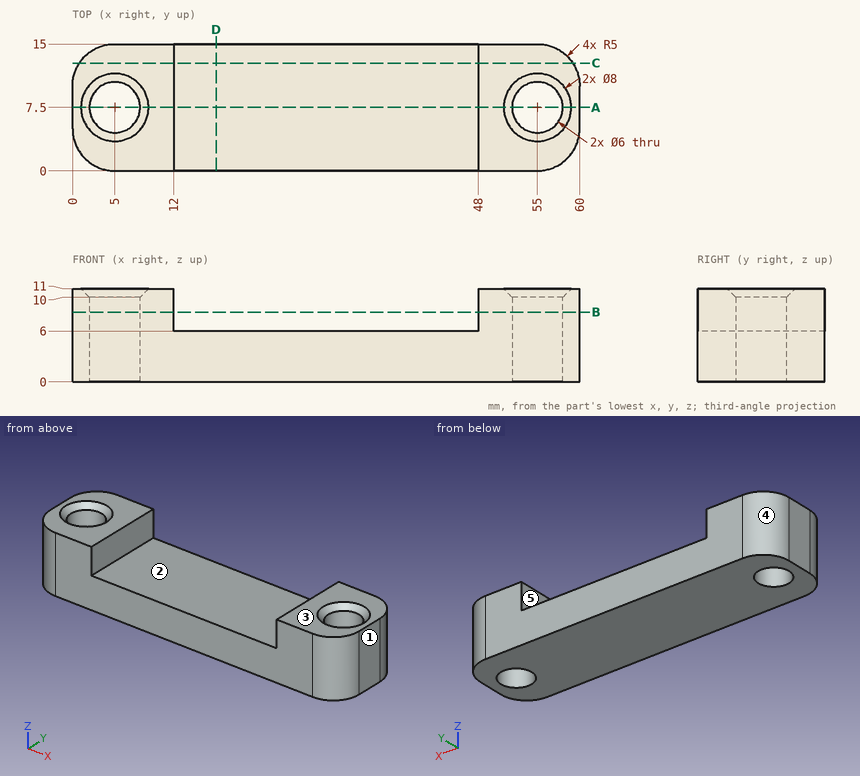
Answer from the drawing. Dimensions are ordinates in mm from the lowest x, y and z of the part. A direction names the side the tool comes from. Coordinates: 2 decimals unless noted, no trailing zeros. Loops run counter-clockwise (first coordinate to the right, second up) from the corner with the lowest first, then second, coordinate; pieces in that order, holes last. Notation, with made-up numbers: (87, -30.5) - (132, -30.5) arc R17 ccw to (132, -24.5) - close; hole circle Ø3 at (-36.75, -26). An arc over 180 degrees is marked (long way). Answer in a Markdown table with one row per item.
1. Find section D-D, the plane x = 17. Write down the section's boundary in (y, z), then the cut area to 3 significant figures.
Conclusion:
| item | result |
|---|---|
| outline | (0, 0) - (15, 0) - (15, 6) - (0, 6) - close |
| area | 90.0 mm² |
2. Find section B-B, the plane z = 8.25. Write down the section's boundary in (x, y), then the cut area to 3 significant figures.
Conclusion:
| item | result |
|---|---|
| outline | (0, 5) arc R5 ccw to (5, 0) - (12, 0) - (12, 15) - (5, 15) arc R5 ccw to (0, 10) - close; (48, 0) - (55, 0) arc R5 ccw to (60, 5) - (60, 10) arc R5 ccw to (55, 15) - (48, 15) - close; hole circle Ø6 at (5, 7.5); hole circle Ø6 at (55, 7.5) |
| area | 282 mm² |
3. Straight lines are drawn through the part: line 1 (X direction, y = 6, z = 7.5); line 2 (Z direction, x = 39.5, y = 1.5); line 3 (X direction, y = 9.5, z = 8). For each, find the intervals that lie inside material, in ascending order.
Conclusion:
| item | result |
|---|---|
| line 1 | x = 0 to 2.4, 7.6 to 12, 48 to 52.4, 57.6 to 60 |
| line 2 | z = 0 to 6 |
| line 3 | x = 0 to 2.76, 7.24 to 12, 48 to 52.76, 57.24 to 60 |
4. Find section C-C, the plane y = 12.75. Write down the section's boundary in (x, z), then the cut area to 3 significant figures.
Conclusion:
| item | result |
|---|---|
| outline | (0.82, 0) - (59.18, 0) - (59.18, 11) - (48, 11) - (48, 6) - (12, 6) - (12, 11) - (0.82, 11) - close |
| area | 462 mm² |
5. Determine the mould class of the marked faces 3, 4 and 5 for opening direction X: +X half, -X half, draft (parallel to the pull), parting line (faces both ways), or undercut.
Conclusion:
| item | result |
|---|---|
| face 3 | draft |
| face 4 | -X half |
| face 5 | undercut |
6. Find section A-A, the plane y = 7.5. Write down the section's boundary in (x, z).
Conclusion:
| item | result |
|---|---|
| outline | (0, 0) - (2, 0) - (2, 10) - (1, 11) - (0, 11) - close; (8, 0) - (52, 0) - (52, 10) - (51, 11) - (48, 11) - (48, 6) - (12, 6) - (12, 11) - (9, 11) - (8, 10) - close; (58, 0) - (60, 0) - (60, 11) - (59, 11) - (58, 10) - close |
7. Given pin 1 (4 mm diameter, centred on x = 45.5, y = 9, fed in from +Z); pin 2 (3 mm diameter, centred on y = 3, z = 6, fed in from -X), each flat-ended and moving along its own axis, determine where each tip first touches the part or whether it passes through.
Conclusion:
| item | result |
|---|---|
| pin 1 | stops at z = 6 |
| pin 2 | stops at x = 0.03 |
8. Which of the six approach directions +Z, -Z, +X, -X, +Y, -Y give full straight-line access (tool end or side, diameter ignored) to the marked faces 1 and 2?
Conclusion:
| item | result |
|---|---|
| face 1 | +Z, -Z, +X, +Y, -Y |
| face 2 | +Z, +Y, -Y |
